Autodesk Inventor part; units mm, degrees
ref_plane "YZ Plane" through (0, 0, 0) normal (1, 0, 0) x (0, 1, 0)
ref_plane "XZ Plane" through (0, 0, 0) normal (0, 1, 0) x (-1, 0, 0)
ref_plane "XY Plane" through (0, 0, 0) normal (0, 0, 1) x (1, 0, 0)
sketch "Эскиз1" plane through (0, 0, 0) normal (0, 1, 0) x (-1, 0, 0)
  line L0 (13.5, -5) -> (-13.5, -5)
  line L1 (-13.5, -5) -> (-13.5, 5)
  line L2 (-13.5, 5) -> (13.5, 5)
  line L3 (13.5, 5) -> (13.5, -5)
  line L4 (-13.5, -5) -> (13.5, 5) construction
  line L5 (13.5, -5) -> (-13.5, 5) construction
  line L6 (-11.5, -3) -> (11.5, -3)
  line L7 (11.5, -3) -> (11.5, 3)
  line L8 (11.5, 3) -> (-11.5, 3)
  line L9 (-11.5, 3) -> (-11.5, -3)
  point P0 (0, 0)
  point P1 (0, 0)
  dimension "d0" = 27
  dimension "d1" = 10
  dimension "d2" = 2
extrude "Выдавливание1" add sketch "Эскиз1" along normal blind 78.4
sketch "Эскиз2" plane through (13.5, 0, 5) normal (1, 0, 0) x (0, 0, -1)
  line L0 (0, 78.4) -> (10, 78.4) construction
  line L1 (10, 78.4) -> (0, 68.4) construction
  line L2 (0, 0) -> (0, 78.4) construction
  line L3 (0, 78.4) -> (10, 68.4) construction
  line L4 (10, 0) -> (10, 78.4) construction
  line L5 (10, 0) -> (0, 10) construction
  line L6 (0, 0) -> (10, 10) construction
  circle A0 centre (5, 73.4) radius 0.5
  circle A1 centre (5, 5) radius 0.5
  point P0 (5, 0)
  dimension "d5" = 1
  dimension "d6" = 1
sketch "Эскиз3" plane through (13.5, 0, -5) normal (0, 0, -1) x (-1, 0, 0)
  line L0 (0, 0) -> (0, 78.4)
  line L1 (27, 0) -> (27, 78.4)
  line L2 (27, 0) -> (27, 78.4)
  line L3 (0, 0) -> (0, 78.4)
  line L4 (0, 78.4) -> (27, 78.4)
  arc A0 (2, 68.4) -> (25, 68.4) centre (13.5, 68.4) ccw
  line L5 (25, 0) -> (25, 78.4)
  line L6 (2, 0) -> (2, 78.4)
  line L7 (25, 0) -> (25, 78.4)
  line L8 (25, 68.4) -> (25, 78.4)
  line L9 (25, 78.4) -> (2, 78.4)
  line L10 (2, 68.4) -> (2, 78.4)
  point P0 (13.5, 0)
  dimension "d10" = 10
extrude "Выдавливание3" cut sketch "Эскиз3" against normal up to surface (2 mm away)
hole "Отверстие1" at (13.5, 73.4, 0) at (13.5, 5, 0) direction (-1, 0, 0) diameter 1 depth 13.5 countersink diameter 1.5 countersink angle 90
mirror "Зеркальное отражение1" about plane through (0, 0, 0) normal (1, 0, 0) of "Отверстие1"
properties part number "board-1-new"
Check sheet for the modelled part. Datum: model origin and axes. Units: mm. A direction names the side the tool comes from. Round coordinates to 2 decimals unless told otherwise and drop trailing zeros. Write each loop counter-clockwise with the first axis right and the second up, starting at its lowest first coordinate (ties: lowest second). Pieces come first, ordered by that corner, then holes. Notation, with made-up numbers: (0, 12.25) - (7, 12.25) arc R32 cw to (7, 44.25) - close; hole circle Ø6 at (74, 35.25). An arc over 180 degrees is marked (long way). Return JSON: item names as keys, results as strings.
Q1. Depth check by flat-ended pin: P1, Ø2, axis at x = 7, y = 64.5, coming from the -Z side. Enter the tip coordinate at first touch or a pass-through.
Returned:
{"P1": "stops at z = 3"}
Q2. Cross-section at D-D (x = -10.25). Record the boundary of the cut face in (y, z).
Returned:
{"outline": "(0, -5) - (63.19, -5) - (63.19, -3) - (0, -3) - close; (0, 3) - (78.4, 3) - (78.4, 5) - (0, 5) - close"}
Q3. Access from +Z, -Z, +X, -X, +Y, -Y to the whole of each face (thin tool, end or side, straight path). Record for faces 1 (the flat face through (0, 26, -3)), 2 (the cylindrical face through (0.253, 56.903, -4.014)), 3 (the flat face through (-13.5, 39, 0)).
Returned:
{"face 1": "+Y, -Y", "face 2": "-Z, +Y", "face 3": "+Z, -Z, -X, +Y, -Y"}
Q4. Cross-section at B-B (x = 7.75). Record the boundary of the cut face in (y, z).
Returned:
{"outline": "(0, -5) - (59.9, -5) - (59.9, -3) - (0, -3) - close; (0, 3) - (78.4, 3) - (78.4, 5) - (0, 5) - close"}
Q5. Cross-section at A-A (y = 17.5). Record the boundary of the cut face in (x, z), then the cut area to 3 significant figures.
Returned:
{"outline": "(-13.5, -5) - (13.5, -5) - (13.5, 5) - (-13.5, 5) - close; hole (-11.5, -3) - (11.5, -3) - (11.5, 3) - (-11.5, 3) - close", "area": "132 mm²"}
Q6. Cross-section at C-C (z = -3.75). Record the boundary of the cut face in (x, y), then the cut area to 3 significant figures.
Returned:
{"outline": "(-13.5, 0) - (13.5, 0) - (13.5, 78.4) - (11.5, 78.4) - (11.5, 68.4) arc R11.5 cw to (-11.5, 68.4) - (-11.5, 78.4) - (-13.5, 78.4) - close", "area": "1,680 mm²"}
Q7. Scan lines: L1, parallel to Y at x = 12, z = 0; L2, parallel to X at y = 47, z = 1.25; L3, parallel to Z at x = -4, y = 12. Record each from-to range of solid material in increasing order. Write a range as from..to.
Returned:
{"L1": "y = 0..4.5, 5.5..72.9, 73.9..78.4", "L2": "x = -13.5..-11.5, 11.5..13.5", "L3": "z = -5..-3, 3..5"}
Q8. Draft check along Z on faces 4 (the flat face through (0, 39, 5)), 5 (the flat face through (0.2, 0, 3.4)), 6 (the flat face through (-11.5, 39, 0)). Enter one of: released by +Z, released by -Z, zero draft, split by the parting line, or undercut.
Returned:
{"face 4": "released by +Z", "face 5": "zero draft", "face 6": "undercut"}
